Geometry: final body of the model. Coordinates: model frame, mm. Face numbers are marked on the shaded views. A direction names the side the tool comes from. Round coordinates to 2 decimals unless told otherwise and drop trailing zeros. Loops run counter-clockwise (first coordinate to the right, second up) from the corner with the lowest first, then second, coordinate; pieces in that order, holes last. Notation, with made-up numbers: M 46.5,-1 L 63.5,-1 A32 cw 63.5,29 Z; hole C 40,-36.5 d5. An arc over 180 degrees is marked long. Answer as a JSON object with one key per item and string values.
from build123d import *

# Parameters (mm, degrees)
MODEL_R             = 3.75005
MODEL_R_2           = 1.300000002
BOSS_EXTRUDE1_DEPTH = 3


with BuildPart() as part:
    # Model → Boss-Extrude1 (new body)
    with BuildSketch(Plane.XY):
        with BuildLine():
            Line((64.397506493, 42.115672183), (58.266368088, 28.207946902))
            ThreePointArc((58.266368088, 28.207946902), (57.851399273, 26.505567789), (58.049287259, 24.764552536))
            ThreePointArc((58.049287259, 24.764552536), (50.559319275, 18.162603648), (50.380520329, 28.145257626))
            ThreePointArc((50.380520329, 28.145257626), (51.799316654, 29.173568367), (52.776187572, 30.6282605))
            Line((52.776187572, 30.6282605), (59.040732097, 45.181361317))
            ThreePointArc((59.040732097, 45.181361317), (63.049082158, 45.972402409), (64.397506493, 42.115672183))
        make_face()
        with Locations((52.777915011, 23.195230557)):
            Circle(MODEL_R, mode=Mode.SUBTRACT)
        with Locations((61.652416233, 43.325828981)):
            Circle(MODEL_R_2, mode=Mode.SUBTRACT)
        with BuildLine():
            Line((59.743787463, 36.517324284), (57.726859465, 31.942173855))
            ThreePointArc((57.726859465, 31.942173855), (56.408443779, 31.430529369), (55.896799293, 32.748945054))
            Line((55.896799293, 32.748945054), (57.913727291, 37.324095484))
            ThreePointArc((57.913727291, 37.324095484), (59.232142977, 37.83573997), (59.743787463, 36.517324284))
        make_face(mode=Mode.SUBTRACT)
    extrude(amount=BOSS_EXTRUDE1_DEPTH)


solid = part.part
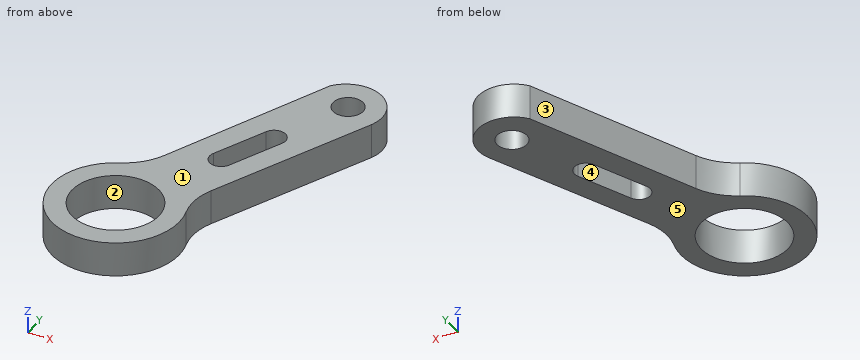
1) Section query A-A (x = 51.5). Return the cut outline in (y, z), and give its area (3 significant figures).
Results:
{"outline": "M 17.85,0 L 19.67,0 L 19.67,3 L 17.85,3 Z; M 26.72,0 L 28.89,0 L 28.89,3 L 26.72,3 Z", "area": "12.0 mm2"}
2) Section query D-D (y = 31). Return the cut outline in (x, z).
Results:
{"outline": "M 52.94,0 L 59.5,0 L 59.5,3 L 52.94,3 Z"}
3) Reachability of the marked faces 4 and 5 from +Z, -Z, +X, -X, +Y, -Y: full face, straight path, thin tool, end or side. Return the list, or none.
Results:
{"face 4": "+Z, -Z", "face 5": "-Z, +X, -X, +Y, -Y"}
4) Pin query (flat end, axial travel): P1, Ø1.5, axis at x = 50, z = 2, coming from the +Y side; P2, Ø1, axis at y = 39, z = 1, coming from the -X side. Return the tip coordinate at first contact, or that it passes through.
Results:
{"P1": "y = 28.34", "P2": "x = 56.16"}
5) Ray query, line 1 (X direction, y = 22.5, z = 0.75); line 2 (Y direction, x = 50.5, z = 2.1); line 3 (Y direction, x = 53, z = 1.3). Return the intervals inside material, ascending.
Results:
{"line 1": "47.32 to 49.09, 56.46 to 58.23", "line 2": "18.19 to 20.22, 26.17 to 28.21", "line 3": "17.7 to 19.45, 26.94 to 31.15"}
6) Section query C-C (z = 1.6). Return the cut outline in (x, y), and give its area (3 significant figures).
Results:
{"outline": "M 50.38,28.15 A5.5 ccw long 58.05,24.76 A5 cw 58.27,28.21 L 64.4,42.12 A3.12 ccw 59.04,45.18 L 52.78,30.63 A5 cw Z; hole C 52.78,23.2 d7.5; hole M 55.9,32.75 A1 ccw 57.73,31.94 L 59.74,36.52 A1 ccw 57.91,37.32 Z; hole C 61.65,43.33 d2.6", "area": "150 mm2"}
7) Section query B-B (y = 42.75). Return the cut outline in (x, z).
Results:
{"outline": "M 57.99,0 L 60.49,0 L 60.49,3 L 57.99,3 Z; M 62.82,0 L 64.57,0 L 64.57,3 L 62.82,3 Z"}
8) Pull-direction query (Y, two-part tool) for the marked faces 1, 2 and 3; classes: +Y half, -Y half, draft (parallel to the pull), parting line (faces both ways), or undercut.
Results:
{"face 1": "draft", "face 2": "undercut", "face 3": "+Y half"}
